The drawing under review shows one solid part. Ordinate dimensions are in mm from its lowest x, y, z. A direction names the side the tool comes from. Give positions to 0.01 mm unless a question says otherwise; leave off trailing zeros. Loops run counter-clockwise (first coordinate to the right, second up) from the corner with the lowest first, then second, coordinate; pieces in that order, holes last. Notation, with made-up numbers: M 32,43 L 78,43 A24 cw 78,56 Z; hole C 0,-25.5 d10. An arc over 180 degrees is marked long. Answer as CSV lines item,"result".
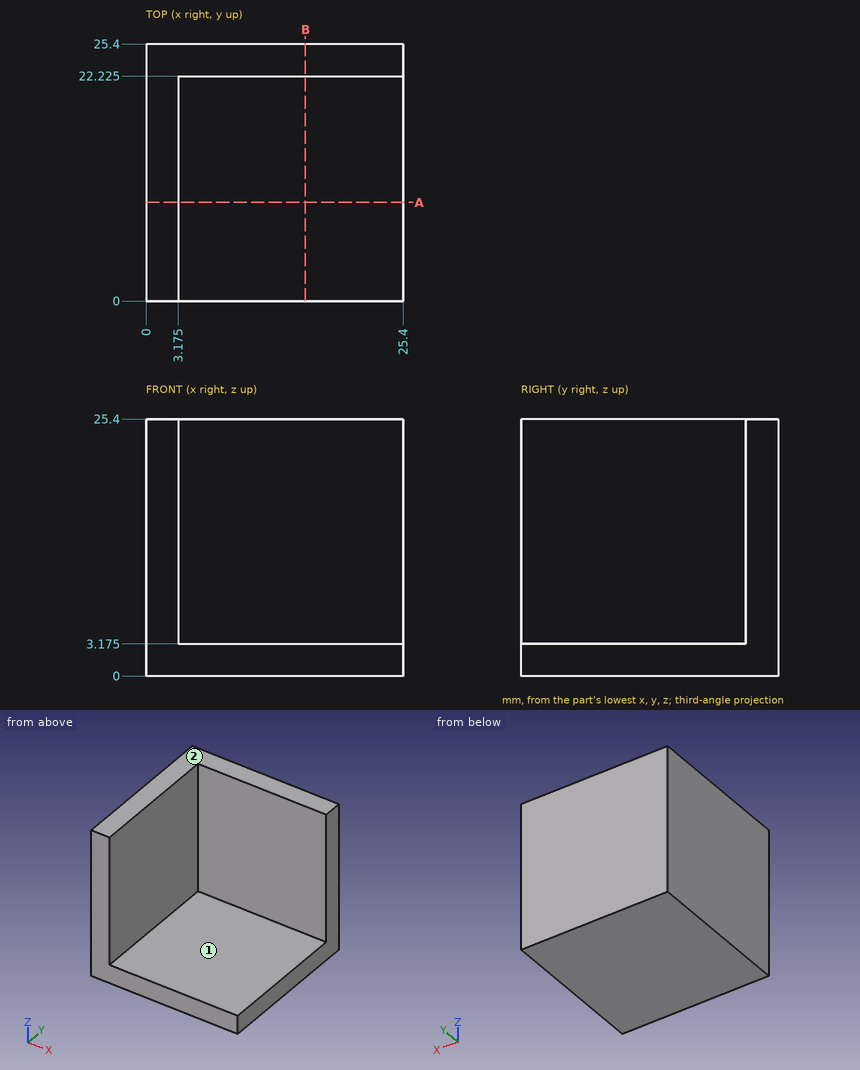
1. For the marked faces 1 and 2, list the 3-axis set-ups (+Z, -Z, +X, -X, +Y, -Y) from which the entire face can be reached by the end or side of a thin tool; tool diameter is ignored.
Answer block:
face 1,"+Z, +X, -Y"
face 2,"+Z, +X, -X, +Y, -Y"
2. To check wall thickness, follow L1, parallel to Z at x = 7.5, y = 20.25 (3 decimals); L2, parallel to Y at x = 7, z = 13.25 (3 decimals). State the ranges of each line that lie inside material, in increasing order. Write a range as [from, to].
Answer block:
L1,"[0, 3.175]"
L2,"[22.225, 25.4]"
3. We need section A-A, the plane y = 9.75. Write out the cut boundary in (x, z) (3 decimals), plus the area to 3 significant figures.
Answer block:
outline,"M 0,0 L 25.4,0 L 25.4,3.175 L 3.175,3.175 L 3.175,25.4 L 0,25.4 Z"
area,"151 mm²"
4. For P1, Ø6.5, axis at y = 10, z = 18.5, coming from the +X side (3 decimals); P2, Ø11, axis at x = 15, y = 15.5, coming from the +Z side (3 decimals); P3, Ø5, axis at x = 8.5, z = 16.5, coming from the -Y side (3 decimals), all flat-tipped, find the tip position at first contact; note any pin that passes through.
Answer block:
P1,"x = 3.175"
P2,"z = 3.175"
P3,"y = 22.225"
5. We need section B-B, the plane x = 15.75. Write out the cut boundary in (y, z) (3 decimals), plus the area to 3 significant figures.
Answer block:
outline,"M 0,0 L 25.4,0 L 25.4,25.4 L 22.225,25.4 L 22.225,3.175 L 0,3.175 Z"
area,"151 mm²"
